```python
from build123d import *

# Parameters (mm, degrees)
SKETCH2_W           = 457.2
SKETCH2_H           = 304.8
BOSS_EXTRUDE1_DEPTH = 3.175
CUT_EXTRUDE1_DEPTH  = 3.175
SKETCH5_R           = 3.175
CUT_EXTRUDE3_DEPTH  = 3.175


with BuildPart() as part:
    # Sketch2 → Boss-Extrude1 (new body)
    with BuildSketch(Plane(origin=(0, 0, 0), x_dir=(1, 0, 0), z_dir=(0, 1, 0))):
        Rectangle(SKETCH2_W, SKETCH2_H)
    extrude(amount=BOSS_EXTRUDE1_DEPTH)

    # Sketch3 → Cut-Extrude1 (cut)
    with BuildSketch(Plane(origin=(0, 3.175, 0), x_dir=(1, 0, 0), z_dir=(0, 1, 0))):
        Polygon((-228.6, -12.7), (-174.955758152, 152.4), (-228.6, 152.4), align=None)
        Polygon((174.955758152, 152.4), (228.6, 152.4), (228.6, -12.7), align=None)
    extrude(amount=-CUT_EXTRUDE1_DEPTH, mode=Mode.SUBTRACT)

    # Sketch5 → Cut-Extrude3 (cut)
    with BuildSketch(Plane(origin=(0, 3.175, 0), x_dir=(1, 0, 0), z_dir=(0, 1, 0))):
        with Locations(Location((0, -114.3, 0), (0, 0, 270))):
            Circle(SKETCH5_R)
        with Locations(Location((0, -76.2, 0), (0, 0, 270))):
            Circle(SKETCH5_R)
        with Locations(Location((0, -38.1, 0), (0, 0, 270))):
            Circle(SKETCH5_R)
    extrude(amount=-CUT_EXTRUDE3_DEPTH, mode=Mode.SUBTRACT)


solid = part.part
```
The model under review builds one solid part; all positions refer to its coordinate system, in mm. Round coordinates to 2 decimals unless told otherwise and drop trailing zeros. Order: outer loops, then holes, each group sorted by start corner. A loop starts at its lowest first (then second) coordinate and runs counter-clockwise, first axis right, second up. Notation, with made-up numbers: (-31, 19.25) - (-16, 19.25) arc R10 cw to (-16, 34.25) - close; hole circle Ø2 at (-36.5, 24.25). An arc over 180 degrees is marked (long way). Answer in a Markdown table with one row per item.
(1) Take a section at C-C on z = -86.5. Write out the cut boundary in (x, y) (3 decimals), plus the area to 3 significant figures.
Result set:
| item | result |
|---|---|
| outline | (-196.368, 0) - (196.368, 0) - (196.368, 3.175) - (-196.368, 3.175) - close |
| area | 1,250 mm2 |
(2) Take a section at B-B on z = -21.5. Write out the cut boundary in (x, y) (3 decimals), plus the area to 3 significant figures.
Result set:
| item | result |
|---|---|
| outline | (-217.488, 0) - (217.488, 0) - (217.488, 3.175) - (-217.488, 3.175) - close |
| area | 1,380 mm2 |
(3) For line 1 (X direction, y = 1.95, z = 114.3) (3 decimals); line 2 (X direction, y = 1.4, z = -62); line 3 (X direction, y = 0.4, z = -110.5), list the stretches that pass through material, from the lowest coordinate up. Write a range as from..to.
Result set:
| item | result |
|---|---|
| line 1 | x = -228.6..-3.175, 3.175..228.6 |
| line 2 | x = -204.33..204.33 |
| line 3 | x = -188.57..188.57 |
(4) Take a section at A-A on y = 2.05. Write out the cut boundary in (x, z) (3 decimals), plus the area to 3 significant figures.
Result set:
| item | result |
|---|---|
| outline | (-228.6, 12.7) - (-174.956, -152.4) - (174.956, -152.4) - (228.6, 12.7) - (228.6, 152.4) - (-228.6, 152.4) - close; hole circle Ø6.35 at (0, 38.1); hole circle Ø6.35 at (0, 76.2); hole circle Ø6.35 at (0, 114.3) |
| area | 130,000 mm2 |
